Source: CAD feature listing. Evaluate the final solid. Frame: model axes, mm. Face numbers are marked on the shaded views. A direction names the side the tool comes from. Round coordinates to 2 decimals unless told otherwise and drop trailing zeros. Write each loop counter-clockwise with the first axis right and the second up, starting at its lowest first coordinate (ties: lowest second). Pieces come first, ordered by that corner, then holes. Notation, with made-up numbers: M 43.5,-9 L 67.5,-9 A12 cw 67.5,1 Z; hole C -5,46.5 d3. An arc over 180 degrees is marked long. Use a Markdown table: item, result.
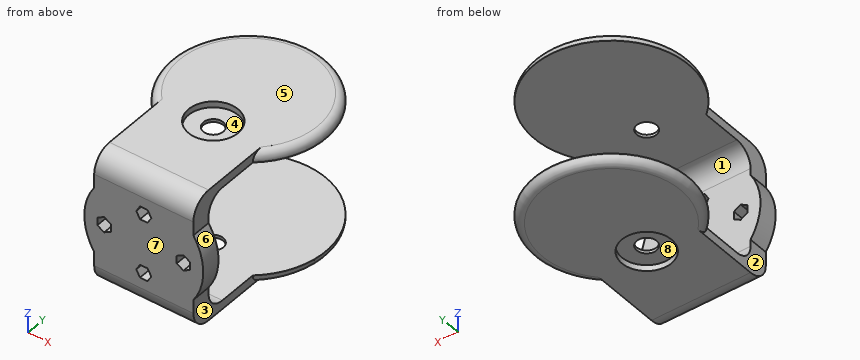
Autodesk Inventor part; units mm, degrees
ref_plane "Work Plane1" through (50, -86.7936, 18.7157) normal (0, 0, -1) x (-1, 0, 0)
ref_plane "YZ Plane" through (0, 0, 0) normal (1, 0, 0) x (0, 1, 0)
ref_plane "XZ Plane" through (0, 0, 0) normal (0, 1, 0) x (-1, 0, 0)
sketch "Sketch1" plane through (0, 0, 0) normal (1, 0, 0) x (0, 1, 0)
  line L0 (-26.7936, -14.7843) -> (-86.7936, -14.7843)
  line L1 (-86.7936, -14.7843) -> (-86.7936, 52.2157)
  line L2 (-86.7936, 52.2157) -> (-26.8407, 52.2157)
  line L3 (-26.8407, 52.2157) -> (-26.7466, 47.7157)
  line L4 (-26.7936, -14.7843) -> (-26.7936, -10.2843)
  line L5 (-26.7936, -10.2843) -> (-76.7936, -10.2843)
  line L6 (-76.7936, -10.2843) -> (-76.7936, 47.7157)
  line L7 (-76.7936, 47.7157) -> (-26.7466, 47.7157)
  point P0 (0, 0)
  point P1 (-26.7936, -12.5343)
  point P2 (-26.7936, 49.9657)
  dimension "d0" = 4.5
  dimension "d1" = 4.5
  dimension "d4" = 60
  dimension "d5" = 50
  dimension "d9" = 58
extrude "Extrusion1" add sketch "Sketch1" along normal blind 50
sketch "Sketch2" plane through (0, -76.7936, 47.7157) normal (0, 1, 0) x (1, 0, 0)
  line L0 (0, 58) -> (0, 0)
  line L1 (0, 0) -> (50, 0)
  line L2 (50, 58) -> (50, 0)
  line L3 (0, 58) -> (50, 58)
  circle A0 centre (25, 29) radius 30
  point P0 (0, 47.7157)
  dimension "d12" = 60
fillet "Fillet1" radius 9 2 edges at (25, -76.7936, -10.2843) (25, -76.7936, 47.7157)
extrude "Extrusion2" add sketch "Sketch2" against normal blind 10 contours A0 L3 L2 L1 L0 | L0 A0 | A0 L3 | L1 A0 | A0 L2
sketch "Sketch4" plane through (0, -86.7936, -14.7843) normal (0, 0, -1) x (-1, 0, 0)
  line L0 (0, 19) -> (0, 60.047)
  line L1 (-50, 59.953) -> (-50, 0)
  line L2 (0, 29.9765) -> (-50, 29.9765)
  circle A0 centre (-25, 68.8186) radius 38.8421
  point P0 (0, 86.7936)
  point P1 (-25, 29.9765)
extrude "Extrusion3" add sketch "Sketch4" against normal blind 4.5 contours A0
fillet "Fillet2" radius 4 1 edges at (25, 20.8671, -14.7843)
ref_plane "Work Plane1" through (50, -86.7936, 18.7157) normal (0, 0, -1) x (-1, 0, 0)
fillet "Fillet3" radius 10 1 edges at (25, -86.7936, -14.7843)
sketch "Sketch6" plane through (0, -86.7936, 52.2157) normal (0, 0, 1) x (1, 0, 0)
  line L0 (0, 39.0913) -> (0, 19)
  line L1 (50, 19) -> (0, 19)
  line L2 (50, 39.0913) -> (50, 19)
  arc A0 (50, 39.0913) -> (0, 39.0913) centre (25, 68.8186) ccw
  circle A1 centre (25, 68.8186) radius 38.8421
  point P0 (0, 86.7936)
extrude "Extrusion4" add sketch "Sketch6" against normal blind 4.5 contours A0 A1
fillet "Fillet4" radius 10 1 edges at (25, -86.7936, 52.2157)
fillet "Fillet5" radius 4 1 edges at (25, 20.8671, 52.2157)
sketch "Sketch7" plane through (25, -17.975, -14.7843) normal (0, 0, -1) x (-1, 0, 0)
  circle A0 centre (0.2258, -22.8186) radius 5
  line L0 (30, -58.8186) -> (25, -58.8186)
  point P0 (25, 17.975)
  dimension "d24" = 36
  dimension "d25" = 10
extrude "Extrusion5" cut sketch "Sketch7" against normal through all
sketch "Sketch8" plane through (25, -17.975, -14.7843) normal (0, 0, -1) x (-1, 0, 0)
  circle A0 centre (0.2258, -22.8186) radius 5
  circle A1 centre (0.2258, -22.8186) radius 12.5
  point P0 (25, 17.975)
  dimension "d28" = 25
extrude "Extrusion6" cut sketch "Sketch8" against normal blind 3
sketch "Sketch9" plane through (0, -76.7936, 52.2157) normal (0, 0, 1) x (1, 0, 0)
  circle A0 centre (24.7742, 36) radius 5
  circle A1 centre (24.7742, 36) radius 12.5
  circle A2 centre (24.7742, 36) radius 12.5
  point P0 (0, 76.7936)
extrude "Extrusion7" cut sketch "Sketch9" against normal blind 3
sketch "Sketch11" plane through (0, -76.7936, 38.7157) normal (0, 1, 0) x (1, 0, 0)
  line L0 (0, 3.4169) -> (0, 0)
  line L1 (50, 0) -> (0, 0)
  line L2 (50, 3.4169) -> (50, 0)
  arc A0 (50, 3.4169) -> (50, 36.5831) centre (25, 20) ccw
  line L3 (50, 40) -> (50, 36.5831)
  line L4 (0, 40) -> (50, 40)
  line L5 (0, 40) -> (0, 36.5831)
  arc A1 (0, 36.5831) -> (0, 3.4169) centre (25, 20) ccw
  line L6 (0, 40) -> (50, 40)
  line L7 (25, 40) -> (25, 0)
  line L8 (-5, 20) -> (55, 20)
  line L9 (26.898, 31.7126) -> (23.102, 31.7126)
  line L10 (23.102, 31.7126) -> (21.204, 35)
  line L11 (21.204, 35) -> (23.102, 38.2874)
  line L12 (23.102, 38.2874) -> (26.898, 38.2874)
  line L13 (26.898, 38.2874) -> (28.796, 35)
  line L14 (28.796, 35) -> (26.898, 31.7126)
  line L15 (48.4075, 18.0327) -> (45, 16.0654)
  line L16 (45, 16.0654) -> (41.5925, 18.0327)
  line L17 (41.5925, 18.0327) -> (41.5925, 21.9673)
  line L18 (41.5925, 21.9673) -> (45, 23.9346)
  line L19 (45, 23.9346) -> (48.4075, 21.9673)
  line L20 (48.4075, 21.9673) -> (48.4075, 18.0327)
  line L21 (26.898, 8.2874) -> (23.102, 8.2874)
  line L22 (23.102, 8.2874) -> (21.204, 5)
  line L23 (21.204, 5) -> (23.102, 1.7126)
  line L24 (23.102, 1.7126) -> (26.898, 1.7126)
  line L25 (26.898, 1.7126) -> (28.796, 5)
  line L26 (28.796, 5) -> (26.898, 8.2874)
  line L27 (1.5925, 18.0327) -> (5, 16.0654)
  line L28 (5, 16.0654) -> (8.4075, 18.0327)
  line L29 (8.4075, 18.0327) -> (8.4075, 21.9673)
  line L30 (8.4075, 21.9673) -> (5, 23.9346)
  line L31 (5, 23.9346) -> (1.5925, 21.9673)
  line L32 (1.5925, 21.9673) -> (1.5925, 18.0327)
  point P0 (0, 38.7157)
  point P1 (25, 35)
  point P2 (25, 20)
  point P3 (45, 20)
  dimension "d43" = 15
  dimension "d44" = 20
extrude "Extrusion9" cut sketch "Sketch11" against normal through all contours L32 L31 L30 L29 L8 | L8 L29 L28 L27 L32 | L24 L23 L22 L21 L7 | L7 L21 L26 L25 L24 | L12 L13 L14 L9 L7 | L7 L9 L10 L11 L12 | L17 L18 L19 L20 L8 | L8 L20 L15 L16 L17
properties part number "task3"
Q1. Mould query, pull axis X, two halves, no side actions, for the marked faces 6, 7 and 8. Classes: +X half, -X half, draft (parallel to the pull), parting line (faces both ways), or undercut.
Results are:
| item | result |
|---|---|
| face 6 | +X half |
| face 7 | draft |
| face 8 | undercut |
Q2. First-contact query: pin 1 Ø8.5 at (y, z) = (-73.5, -7) entering from -X; pin 2 Ø1.9 at (x, y) = (25.5, -80) entering from -Z; pin 3 Ø18.5 at (y, z) = (-58, -3.5) entering from +X. Flat tips, straight axial feed; report the tip coordinate or a pass-through.
Results are:
| item | result |
|---|---|
| pin 1 | x = 0 |
| pin 2 | z = -14.53 |
| pin 3 | x = 50 |
Q3. Section A-A on x = -2.5. Give the number of separate pieces and of enclosed holes in the cut face, plus the area to 3 significant figures.
Results are:
| item | result |
|---|---|
| separate pieces | 3 |
| enclosed holes | 0 |
| area | 714 mm^2 |
Q4. Reachability of the marked faces 1, 2, 3, 4 and 5 from +Z, -Z, +X, -X, +Y, -Y: full face, straight path, thin tool, end or side. Return the list, or none.
Results are:
| item | result |
|---|---|
| face 1 | +X, -X, +Y |
| face 2 | -Z, -X, -Y |
| face 3 | -Z, +X, -Y |
| face 4 | +Z |
| face 5 | +Z, +X, -X, +Y, -Y |
Q5. Line query: L1, parallel to Z at x = 33, y = 13.5; L2, parallel to Y at x = 6, z = 11; L3, parallel to Z at x = 39, y = -69. Output: solid intervals per line, ascending.
Results are:
| item | result |
|---|---|
| L1 | -14.78 to -10.28, 47.72 to 52.22 |
| L2 | -86.79 to -76.79 |
| L3 | -14.78 to -10.2, 47.63 to 52.22 |
Q6. Section B-B on z = 27.5. Return loops of the section in (x, y).
Results are:
| item | result |
|---|---|
| outline | M -3.69,-86.79 L 53.69,-86.79 L 53.69,-76.79 L -3.69,-76.79 Z |
